from build123d import *

# Parameters (mm, degrees)
F0_W     = 715
F0_H     = 75
F1_DEPTH = 75
F2_R     = 10
F3_T     = -5


with BuildPart() as f1:
    # F0 (on Front) → F1 (new body)
    with BuildSketch(Plane.XZ):
        with Locations((-357.5, 37.5)):
            Rectangle(F0_W, F0_H)
    extrude(amount=-F1_DEPTH)

    # F2
    f2_edges = [f1.edges().sort_by_distance(p)[0] for p in [
        (-357.5, 0, 0),
    ]]
    fillet(f2_edges, radius=F2_R)

    # F3
    f3_openings = [f1.faces().sort_by_distance(p)[0] for p in [
        (-357.5, 37.5, 75),
        (-357.5, 75, 37.5),
        (0, 37.635061, 37.635061),
        (-715, 37.635061, 37.635061),
    ]]
    offset(amount=F3_T, openings=f3_openings)


solid = f1.part
Source: CAD feature listing. Evaluate the final solid. Frame: model axes, mm. A direction names the side the tool comes from. Coordinates: 2 decimals unless noted, no trailing zeros. Loops run counter-clockwise (first coordinate to the right, second up) from the corner with the lowest first, then second, coordinate; pieces in that order, holes last. Notation, with made-up numbers: (0.5, 66.5) -> (31.5, 66.5) arc R21 cw to (31.5, 92.5) -> close; hole circle Ø1 at (21.25, -35.75). An arc over 180 degrees is marked (long way). Answer in a Markdown table with one row per item. Add a question column.
Q1. Contact query for flat-ended pins moving along their axis: pin 1 Ø4 at (x, y) = (-244.5, 21) entering from +Z; pin 2 Ø3 at (x, z) = (-445.5, 62.5) entering from +Y. Output: stop coordinate, or through.
Q2. Section A-A on x = -328. Return the cut outline in (y, z).
Q3. Section B-B on y = 56.5. Return the cut outline in (x, z).
Q4. Reachability of faces 1 (the face through (0, 21, 4)), 2 (the face through (-363, 5, 43)) from +Z, -Z, +X, -X, +Y, -Y: full face, straight path, thin tool, end or side. Return the list, or none.
Q5. Ray query, line 1 along Y through (x, z) = (-522, 26.5); line 2 along Y through (x, z) = (-73.5, 6). Return the intervals inside material, ascending.
Computed values:
| question | item | result |
|---|---|---|
| 1 | pin 1 | stops at z = 5 |
| 1 | pin 2 | stops at y = 5 |
| 2 | outline | (0, 10) arc R10 ccw to (10, 0) -> (75, 0) -> (75, 5) -> (10, 5) arc R5 cw to (5, 10) -> (5, 75) -> (0, 75) -> close |
| 3 | outline | (-715, 0) -> (0, 0) -> (0, 5) -> (-715, 5) -> close |
| 4 | face 1 | +Z, -Z, +X, +Y, -Y |
| 4 | face 2 | +Z, +X, -X, +Y |
| 5 | line 1 | y = 0 to 5 |
| 5 | line 2 | y = 0.83 to 7 |
